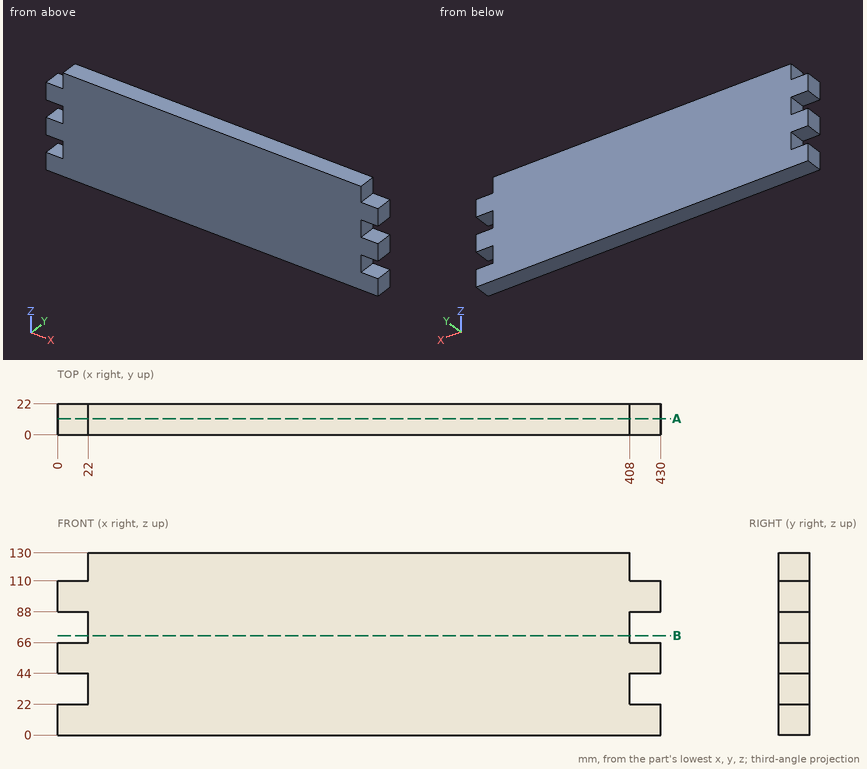
Geometry check sheet. Reference: drawing and pictorial views, mm from the part's lowest x, y, z. Give positions to 0.01 mm unless a question says otherwise; leave off trailing zeros. Order: outer loops, then holes, each group sorted by start corner. A loop starts at its lowest first (then second) coordinate and runs counter-clockwise, first axis right, second up.
1. Section check A-A, the plane y = 11.5. Enter the section's corners in (x, z), and give its area (3 significant figures).
2. Thickness scan on L1, parallel to X at y = 17.5, z = 42.5. Record the ranges inside material, lowest first.
3. Section check B-B, the plane z = 71. Enter the section's corners in (x, y).
4. Gauge pin test, flat ends, axial feed: pin 1 Ø11 at (x, y) = (14.5, 7) entering from +Z; pin 2 Ø6 at (x, y) = (249, 4.5) entering from -Z; pin 3 Ø10 at (y, z) = (6.5, 121.5) entering from +X; pin 4 Ø6.5 at (y, z) = (10.5, 72) entering from -X. Record the tip position at first contact, or that the pin passes through.
Values follow:
1. outline: (0, 0) - (430, 0) - (430, 22) - (408, 22) - (408, 44) - (430, 44) - (430, 66) - (408, 66) - (408, 88) - (430, 88) - (430, 110) - (408, 110) - (408, 130) - (22, 130) - (22, 110) - (0, 110) - (0, 88) - (22, 88) - (22, 66) - (0, 66) - (0, 44) - (22, 44) - (22, 22) - (0, 22) - close
1. area: 53,100 mm2
2. L1: x = 22 to 408
3. outline: (22, 0) - (408, 0) - (408, 22) - (22, 22) - close
4. pin 1: stops at z = 110
4. pin 2: stops at z = 0
4. pin 3: stops at x = 408
4. pin 4: stops at x = 22
